```python
from build123d import *

# Parameters (mm, degrees)
F1_DEPTH = 63.5
F0_W     = 25.4
F0_H     = 19.05
F2_DEPTH = 25.4
F3_DEPTH = 7.9375
F5_R     = 6.35


with BuildPart() as f1:
    # F0 (on Front) → F1 (new body, symmetric)
    with BuildSketch(Plane.XZ):
        Polygon((22.225, 9.525), (-41.275, 9.525), (-41.275, -9.525), (41.275, -9.525), (41.275, 9.525), align=None)
    extrude(amount=F1_DEPTH, both=True)

    # F0 (on Front) → F2 (join, symmetric)
    with BuildSketch(Plane.XZ):
        with BuildLine():
            Line((22.225, 27.0002), (22.225, 9.525))
            Line((22.225, 9.525), (41.275, 9.525))
            Line((41.275, 9.525), (41.275, 27.0002))
            ThreePointArc((41.275, 27.0002), (45.9246798487, 38.2255201513), (57.15, 42.8752))
            Line((57.15, 42.8752), (60.325, 42.8752))
            Line((60.325, 42.8752), (60.325, 61.9252))
            Line((60.325, 61.9252), (57.15, 61.9252))
            add(Edge.make_bspline(
                [(55.0505614157, 61.8620413546), (55.7553301677, 61.8927275326), (56.4552712622, 61.9138638229), (57.15, 61.9252)],
                knots=[109.5945481274, 109.5945481274, 109.5945481274, 109.5945481274, 111.5045361635, 111.5045361635, 111.5045361635, 111.5045361635], degree=3))
            ThreePointArc((55.0505614157, 61.8620413546), (31.7228637323, 50.9421373949), (22.225, 27.0002))
        make_face()
        with Locations((73.025, 52.4002)):
            Rectangle(F0_W, F0_H)
    extrude(amount=F2_DEPTH, both=True)

    # F0 (on Front) → F3 (join, symmetric)
    with BuildSketch(Plane.XZ):
        with BuildLine():
            add(Edge.make_bspline(
                [(-41.275, 9.525), (-41.7230096013, 26.8981728719), (14.611139049, 60.1012775438), (55.0505614157, 61.8620413546)],
                knots=[0, 0, 0, 0, 109.5945481274, 109.5945481274, 109.5945481274, 109.5945481274], degree=3))
            Line((-41.275, 9.525), (22.225, 9.525))
            Line((22.225, 9.525), (22.225, 27.0002))
            ThreePointArc((22.225, 27.0002), (31.7228637323, 50.9421373949), (55.0505614157, 61.8620413546))
        make_face()
    extrude(amount=F3_DEPTH, both=True)

    # F0 (on Front) → F4 (revolve)
    with BuildSketch(Plane.XZ):
        Polygon((85.725, 66.675), (85.725, 61.9252), (85.725, 42.8752), (85.725, 34.925), (111.125, 34.925), (111.125, 66.675), align=None)
    revolve(axis=Axis((85.725, 0, 50.8), (0, 0, 1)))

    # F5
    f5_edges = [f1.edges().sort_by_distance(p)[0] for p in [
        (-41.275, -63.5, 0),
        (41.275, -63.5, 0),
        (41.275, 63.5, 0),
        (-41.275, 63.5, 0),
    ]]
    fillet(f5_edges, radius=F5_R)


solid = f1.part
```
Part model, mm, in its own coordinate system. A direction names the side the tool comes from. Round coordinates to 2 decimals unless told otherwise and drop trailing zeros. Loops run counter-clockwise (first coordinate to the right, second up) from the corner with the lowest first, then second, coordinate; pieces in that order, holes last. Notation, with made-up numbers: (22.25, 19) -> (73.25, 19) arc R6 ccw to (73.25, 26) -> close; hole circle Ø7 at (47, 59.25). An arc over 180 degrees is marked (long way). Use a Markdown table: item, result.
1) Probe line 1 (X direction, y = -38.5, z = 2) (3 decimals); line 2 (Z direction, x = -5, y = 24) (3 decimals); line 3 (Y direction, x = 3, z = 29). List the from-to ranges inside material, lowest first. Write a range as [from, to].
The answers:
| item | result |
|---|---|
| line 1 | x = [-41.275, 41.275] |
| line 2 | z = [-9.525, 9.525] |
| line 3 | y = [-7.94, 7.94] |
2) Cut at B-B, the plane y = 33. List the corners of the cut face in (x, z) (3 decimals), and give its area (3 significant figures).
The answers:
| item | result |
|---|---|
| outline | (-41.275, -9.525) -> (41.275, -9.525) -> (41.275, 9.525) -> (-41.275, 9.525) -> close |
| area | 1,570 mm2 |
3) Cut at A-A, the plane z = 2.5. List the corners of the cut face in (x, y) (3 decimals).
The answers:
| item | result |
|---|---|
| outline | (-41.275, -57.15) arc R6.35 ccw to (-34.925, -63.5) -> (34.925, -63.5) arc R6.35 ccw to (41.275, -57.15) -> (41.275, 57.15) arc R6.35 ccw to (34.925, 63.5) -> (-34.925, 63.5) arc R6.35 ccw to (-41.275, 57.15) -> close |
4) Drop flat-ended pins along their axis: pin 1 Ø3 at (y, z) = (-6, 0) entering from -X (3 decimals); pin 2 Ø1.5 at (x, y) = (90, 6) entering from -Z (3 decimals); pin 3 Ø15.5 at (x, z) = (52.5, 28) entering from -Y; pin 4 Ø5 at (x, z) = (70, 40) entering from -Y. Give the stop position or say it passes through.
The answers:
| item | result |
|---|---|
| pin 1 | stops at x = -41.275 |
| pin 2 | stops at z = 34.925 |
| pin 3 | passes through |
| pin 4 | stops at y = -21.69 |
5) Tool access for faces 1 (the flat face through (60, 2, 42.875)), 2 (the flat face through (-3, -7.938, 30)), 3 (the flat face through (60, -2, 61.925)), 4 (the cylindrical face through (31.98, 16.55, 51.21)), 5 (the flat face through (41.275, -1, 4)): list every direction of +Z, -Z, +X, -X, +Y, -Y with a clear straight run to the whole face (end or side of a thin tool).
The answers:
| item | result |
|---|---|
| face 1 | -Z |
| face 2 | +Z, -X, -Y |
| face 3 | +Z, -X |
| face 4 | +Z, -X, +Y |
| face 5 | -Z, +X, +Y, -Y |
